Can you work these out from the model? Positions are in its coordinate system, mm. A direction names the side the tool comes from. Round coordinates to 2 decimals unless told otherwise and drop trailing zeros. Order: outer loops, then holes, each group sorted by start corner. A loop starts at its lowest first (then second) coordinate and runs counter-clockwise, first axis right, second up. Notation, with made-up numbers: M -28.75,84 L -20.75,84 A8 ccw -20.75,90 Z; hole C 54.25,41 d5. An arc over 180 degrees is marked long. One line per question, with ' | ' between items.
```python
from build123d import *

# Parameters (mm, degrees)
F1_DEPTH = 3.125
F2_W     = 6
F2_H     = 50
F2_W_2   = 50
F2_H_2   = 6
F3_DEPTH = 2
F4_R     = 2.7
F5_DEPTH = 25
F6_R     = 2
F8_DEPTH = 25
F9_R     = 2


# Not quite as in the source:
# - a feature names something its author has since deleted; it is built from what else it names


with BuildPart() as f1:
    # F0 (on Top) → F1 (new body)
    with BuildSketch(Plane.XY):
        with BuildLine():
            Line((35, 35), (15, 35))
            ThreePointArc((15, 35), (-4.5539513718, 4.5539513718), (-35, -15))
            Line((-35, -15), (-35, -35))
            Line((-35, -35), (35, -35))
            Line((35, -35), (35, 35))
        make_face()
    extrude(amount=F1_DEPTH)

    # F2 (on face) → F3 (join)
    with BuildSketch(Plane(origin=(0, 0, 0), x_dir=(1, 0, 0), z_dir=(0, 0, -1))):
        with Locations((25, -10)):
            Rectangle(F2_W, F2_H)
        with Locations((-10, 25)):
            Rectangle(F2_W_2, F2_H_2)
    extrude(amount=F3_DEPTH)

    # F4 (on face) → F5 (cut)
    with BuildSketch(Plane(origin=(0, 0, -2), x_dir=(1, 0, 0), z_dir=(0, 0, -1))):
        with Locations((25, -25)):
            Circle(F4_R)
        with Locations((25, 5)):
            Circle(F4_R)
        with Locations((5, 25)):
            Circle(F4_R)
        with Locations((-25, 25)):
            Circle(F4_R)
    extrude(amount=-F5_DEPTH, mode=Mode.SUBTRACT)

    # F6
    f6_edges = [f1.edges().sort_by_distance(p)[0] for p in [
        (35, 35, 1.5625),
        (15, 35, 1.5625),
        (-35, -15, 1.5625),
        (-35, -35, 1.5625),
        (35, -35, 1.5625),
    ]]
    fillet(f6_edges, radius=F6_R)

    # F7 (on Top) → F8 (cut)
    with BuildSketch(Plane.XY):
        with BuildLine():
            Line((15, -10.0502525317), (15, 20))
            ThreePointArc((15, 20), (9.1151461726, 10.9887424757), (2.2488038315, 2.7009436368))
            Line((2.2488038315, 2.7009436368), (15, -10.0502525317))
        make_face()
        with BuildLine():
            ThreePointArc((-2.7009436368, -2.2488038315), (-10.9887424757, -9.1151461726), (-20, -15))
            Line((-20, -15), (10.0502525317, -15))
            Line((10.0502525317, -15), (-2.7009436368, -2.2488038315))
        make_face()
    extrude(amount=F8_DEPTH, mode=Mode.SUBTRACT)

    # F9
    f9_edges = [f1.edges().sort_by_distance(p)[0] for p in [
        (15, 20, 1.5625),
        (-20, -15, 1.5625),
        (10.050253, -15, 1.5625),
        (15, -10.050253, 1.5625),
    ]]
    fillet(f9_edges, radius=F9_R)


solid = f1.part
```
(1) If we section it at C-C on x = 12.5: Please give me the cut outline in (y, z) (3 decimals).
Final values:
outline: M -35,0 L -28,0 L -28,-2 L -22,-2 L -22,0 L -7.158,0 L -7.158,3.125 L -35,3.125 Z; M 14.96,0 L 28.998,0 L 28.998,3.125 L 14.96,3.125 Z
(2) Please list where these lines run through material, in increasing order: probe 1 along Y at (x, z) = (25, 0.4); probe 2 along X at (y, z) = (-25, -0.95); probe 3 along X at (y, z) = (-25, 1.8). Write a range as [from, to].
Final values:
probe 1: [-35, -7.7], [-2.3, 22.3], [27.7, 35] | probe 2: [-35, -27.7], [-22.3, 2.3], [7.7, 15] | probe 3: [-35, -27.7], [-22.3, 2.3], [7.7, 35]
(3) If we section it at A-A on x = 25: Please give me the cut outline in (y, z) (3 decimals), plus the area to 3 significant figures.
Final values:
outline: M -35,0 L -15,0 L -15,-2 L -7.7,-2 L -7.7,3.125 L -35,3.125 Z; M -2.3,-2 L 22.3,-2 L 22.3,3.125 L -2.3,3.125 Z; M 27.7,-2 L 35,-2 L 35,3.125 L 27.7,3.125 Z | area: 263 mm^2
(4) Thinking about a two-plate mould opening in X: for faces 4 (the flat face through (15, -25, -1)), 5 (the cylindrical face through (-14.946, -13.552, 1.584)), 6 (the flat face through (-35, -25, 1)), which applies, released by +X, released by -X, zero draft, split by the parting line, or undercut?
Final values:
face 4: released by +X | face 5: undercut | face 6: released by -X
(5) Will these pins go through, and if not, where does the flat tip stop? pin 1 Ø3 at (x, y) = (25, 25) entering from +Z; pin 2 Ø1.5 at (x, z) = (-27.5, 0) entering from +Y; pin 3 Ø12 at (x, y) = (-2, -7) entering from +Z (3 decimals); pin 4 Ø1.6 at (x, z) = (24, -1) entering from -Y.
Final values:
pin 1: through | pin 2: y = -11.42 | pin 3: z = 3.125 | pin 4: y = -15
(6) On a 3-axis mill with a long thin cutter (end or side, diameter ignored), from which of +Z, -Z, +X, -X, +Y, -Y can I reach the whole of each face in a straight line? I mean faces 1 (the flat face through (22, 10, -1)), 2 (the flat face through (7, -7, 0)), 3 (the cylindrical face through (7.057, -13.796, 1.584)). Say none if no direction works.
Final values:
face 1: -Z, -X, +Y, -Y | face 2: -Z | face 3: +Z, -Z
(7) If we section it at B-B on y = 4: Please give me the cut outline in (x, z) (3 decimals).
Final values:
outline: M -5.113,0 L 3.433,0 L 3.433,3.125 L -5.113,3.125 Z; M 15,0 L 22,0 L 22,-2 L 28,-2 L 28,0 L 35,0 L 35,3.125 L 15,3.125 Z
